Model file for the job. Use its own axes, mm. A direction names the side the tool comes from. Give positions to 0.01 mm unless a question says otherwise; leave off trailing zeros. Write each loop counter-clockwise with the first axis right and the second up, starting at its lowest first coordinate (ties: lowest second). Pieces come first, ordered by that corner, then holes. Notation, with made-up numbers: (18, 81) - (23, 81) arc R22 ccw to (23, 97) - close; hole circle Ø3 at (-38.75, 77). An arc over 180 degrees is marked (long way). Use a Markdown table: item, result. Add a question column.
```python
from build123d import *

# Parameters (mm, degrees)
F0_W     = 127
F0_H     = 127
F0_R     = 50.8
F1_DEPTH = 63.5
F2_DEPTH = 12.7


with BuildPart() as f1:
    # F0 (on Front) → F1 (new body, symmetric)
    with BuildSketch(Plane.XZ):
        Rectangle(F0_W, F0_H)
        Circle(F0_R, mode=Mode.SUBTRACT)
    extrude(amount=F1_DEPTH, both=True)

    # F0 (on Front) → F2 (join, symmetric)
    with BuildSketch(Plane.XZ):
        Circle(F0_R)
    extrude(amount=F2_DEPTH, both=True)


solid = f1.part
```
(1) Probe probe 1 along Z at (x, y) = (0, 29.5); probe 2 along Y at (x, z) = (-37, 20.5); probe 3 along X at (y, z) = (-19.5, 13). List the from-to ranges inside material, lowest first. Write a range as [from, to].
(2) Which spindle directions (+Z, -Z, +X, -X, +Y, -Y) get a long thin tool onto all of the face, cutting with end or side? Do faces 1 (the cylindrical face through (-11.012, 38.456, -49.592)), 2 (the flat face through (-43, 63.5, 29)), 3 (the cylindrical face through (-11.012, -37.744, -49.592)). Say none if no direction does.
(3) Band-saw the part on A-A (x = 0). Write the cut outline in (y, z).
(4) Band-saw the part on B-B (y = -28.5). Write the cut outline in (x, z).
(5) Band-saw the part on C-C (z = 0). Write the cut outline in (x, y), then the cut area to 3 significant figures.
(6) Two-plate mould, pull along X, no slides. Class faces 4 (the flat face through (63.5, -1, -1)), 5 (the flat face through (-1, -12.7, 1)), 6 (the flat face through (-63.5, -1, -1)), 7 (the flat face through (-1, -1, 63.5)): +X half, -X half, draft (parallel to the pull), parting line (faces both ways), or undercut.
(7) Flat gauge pins, fed straight in: pin 1 (8 mm diameter, centred on x = -23.5, z = 12.5, fed in from -Y); pin 2 (1 mm diameter, centred on x = -12.5, z = 13, fed in from +Y). Where does each tip first touch, or does it go through?
Model answer:
| question | item | result |
|---|---|---|
| 1 | probe 1 | z = [-63.5, -50.8], [50.8, 63.5] |
| 1 | probe 2 | y = [-12.7, 12.7] |
| 1 | probe 3 | x = [-63.5, -49.11], [49.11, 63.5] |
| 2 | face 1 | +Y |
| 2 | face 2 | +Z, -Z, +X, -X, +Y |
| 2 | face 3 | -Y |
| 3 | outline | (-63.5, -63.5) - (63.5, -63.5) - (63.5, -50.8) - (12.7, -50.8) - (12.7, 50.8) - (63.5, 50.8) - (63.5, 63.5) - (-63.5, 63.5) - (-63.5, 50.8) - (-12.7, 50.8) - (-12.7, -50.8) - (-63.5, -50.8) - close |
| 4 | outline | (-63.5, -63.5) - (63.5, -63.5) - (63.5, 63.5) - (-63.5, 63.5) - close; hole circle Ø101.6 at (0, 0) |
| 5 | outline | (-63.5, -63.5) - (-50.8, -63.5) - (-50.8, -12.7) - (50.8, -12.7) - (50.8, -63.5) - (63.5, -63.5) - (63.5, 63.5) - (50.8, 63.5) - (50.8, 12.7) - (-50.8, 12.7) - (-50.8, 63.5) - (-63.5, 63.5) - close |
| 5 | area | 5,810 mm^2 |
| 6 | face 4 | +X half |
| 6 | face 5 | undercut |
| 6 | face 6 | -X half |
| 6 | face 7 | draft |
| 7 | pin 1 | stops at y = -12.7 |
| 7 | pin 2 | stops at y = 12.7 |
